Check sheet for the modelled part. Datum: model origin and axes. Units: mm. A direction names the side the tool comes from. Give positions to 0.01 mm unless a question says otherwise; leave off trailing zeros. Loops run counter-clockwise (first coordinate to the right, second up) from the corner with the lowest first, then second, coordinate; pieces in that order, holes last. Notation, with made-up numbers: M 8.5,-39.5 L 66.5,-39.5 A15 cw 66.5,-35.5 Z; hole C -30.5,-16.5 d10. An arc over 180 degrees is marked long. Write each question's results on one line, items separated by ' | '. Start each with the question number.
1. Sectioned sample at B-B on z = -2.75. Record the cut outline in (x, y).
2. Go/stop test with flat-tipped pins: pin 1 (5 mm diameter, centred on x = 10.5, y = 6.5, fed in from +Z); pin 2 (2 mm diameter, centred on y = 6.5, z = -3.5, fed in from +X); pin 3 (4 mm diameter, centred on x = 7, y = 3, fed in from -Z). Record where each tip stops, or that it passes through.
3. Material ranges on line 1 along Y through (x, z) = (11, -9.5); line 2 along X through (y, z) = (3, -3.5); line 3 along Z through (x, y) = (4.25, 7.25), recorded low to high.
4. Sectioned sample at C-C on x = 1.5. Record the cut outline in (y, z), and give its area (3 significant figures).
5. Tool access check on faces 1 (the cylindrical face through (11.437, 5.084, -11.189)), 2 (the cylindrical face through (4, 5, -3)). Record the directions out of +Z, -Z, +X, -X, +Y, -Y that give a thin tool (end or side, any length) a straight path to the whole face; none if there is none.
6. Sectioned sample at A-A on y = 7. Record the cut outline in (x, z).
7. Sectioned sample at D-D on z = -5.25. Record the cut outline in (x, y), and give its area (3 significant figures).
8. Draft check along Z on faces 3 (the flat face through (8, 10, -8)), 4 (the cylindrical face through (2.859, 5.084, -2.797)), 5 (the flat face through (8, 11, -8)). Enter one of: pulls with the +Z half, pulls with the -Z half, needs draft (parallel to the pull), parting line crosses it, or undercut.
```python
from build123d import *

# Parameters (mm, degrees)
SKETCH_1_W          = 12
SKETCH_1_H          = 12
SKETCH_1_W_2        = 10
SKETCH_1_H_2        = 10
THINREVOLVE90_ANGLE = 90


with BuildPart() as part:
    # 草图1 → ThinRevolve90 (revolve)
    with BuildSketch(Plane.XY):
        with Locations((10, 5)):
            Rectangle(SKETCH_1_W, SKETCH_1_H)
        with Locations((10, 5)):
            Rectangle(SKETCH_1_W_2, SKETCH_1_H_2, mode=Mode.SUBTRACT)
    revolve(axis=Axis((0, 0, 0), (0, 1, 0)), revolution_arc=THINREVOLVE90_ANGLE)


solid = part.part
```
Output values:
1) outline: M 2.9,-1 L 15.76,-1 L 15.76,11 L 2.9,11 Z; hole M 4.18,0 L 14.75,0 L 14.75,10 L 4.18,10 Z
2) pin 1: z = -7.48 | pin 2: x = 15.8 | pin 3: z = -15.2
3) line 1: -1 to 0, 10 to 11 | line 2: 1.94 to 3.57, 14.59 to 15.61 | line 3: -15.43 to -14.39, -2.63 to 0
4) outline: M -1,-15.93 L 11,-15.93 L 11,-3.71 L -1,-3.71 Z; hole M 0,-14.92 L 10,-14.92 L 10,-4.77 L 0,-4.77 Z | area: 45.1 mm2
5) face 1: -Z, +X, +Y, -Y | face 2: none
6) outline: M 0,-16 A16 ccw 16,0 L 15,0 A15 cw 0,-15 Z; M 0,-5 A5 ccw 5,0 L 4,0 A4 cw 0,-4 Z
7) outline: M 0,-1 L 15.11,-1 L 15.11,11 L 0,11 L 0,10 L 14.05,10 L 14.05,0 L 0,0 Z | area: 40.9 mm2
8) face 3: undercut | face 4: pulls with the +Z half | face 5: needs draft
